Input: part model. Units: mm. Frame: model coordinates. Face numbers are marked on the shaded views. A direction names the side the tool comes from. Coordinates: 2 decimals unless noted, no trailing zeros. Loops run counter-clockwise (first coordinate to the right, second up) from the corner with the lowest first, then second, coordinate; pieces in that order, holes last.
Item 1: Pull-direction query (X, two-part tool) for the marked faces 1, 2, 3 and 4; classes: released by +X, released by -X, zero draft, split by the parting line, or undercut.
Item 2: Section C-C on x = -6. Return loops of the section in (y, z).
Item 3: Contact query for flat-ended pins moving along their axis: P1, Ø6, axis at x = 28.5, y = -37, coming from the -Z side; P2, Ø3, axis at x = -7.5, z = 42, coming from the +Y side. Output: stop coordinate, or through.
Item 4: Reachability of the marked faces 5 and 6 from +Z, -Z, +X, -X, +Y, -Y: full face, straight path, thin tool, end or side. Return the list, or none.
Item 5: Section B-B on y = 11.5. Return loops of the section in (x, z).
Item 6: Ray query, line 1 along X through (y, z) = (11.5, 58); line 2 along Y through (x, z) = (45, 51); line 3 along Z through (x, y) = (5.5, 21). Return the intervals inside material, ascending.
Item 7: Section A-A on z = 19.5. Return loops of the section in (x, y), and give its area (3 significant figures).
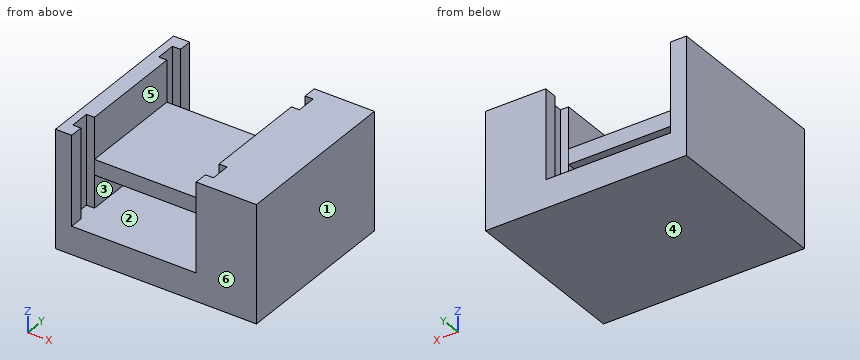
```python
from build123d import *

# Parameters (mm, degrees)
F1_DEPTH  = 17.93161
F2_DEPTH  = 75.24566
F3_W      = 80
F3_H      = 9.859875
F4_DEPTH  = 33.73
F2_FACE_W = 110
F2_FACE_H = 75.24566
F5_DEPTH  = 28.33094


with BuildPart() as f1:
    # F0 (on Top) → F1 (new body)
    with BuildSketch(Plane.XY):
        Polygon((-40, -55), (0, -55), (0, 0), (-40, 0), (-40, -33.72997), (-45.169481, -33.72997), (-45.169481, -46.42997), (-40, -46.42997), align=None)
        Polygon((0, 0), (0, -55), (40, -55), (40, -46.42997), (45.169481, -46.42997), (45.169481, -33.72997), (40, -33.72997), (40, 0), align=None)
        Polygon((-40, 0), (0, 0), (0, 55), (-40, 55), (-40, 46.42997), (-45.169481, 46.42997), (-45.169481, 33.72997), (-40, 33.72997), align=None)
        Polygon((0, 55), (0, 0), (40, 0), (40, 33.72997), (45.169481, 33.72997), (45.169481, 46.42997), (40, 46.42997), (40, 55), align=None)
        Polygon((-50.338964, -55), (-40, -55), (-40, -46.42997), (-45.169481, -46.42997), (-45.169481, -33.72997), (-40, -33.72997), (-40, 0), (-50.338964, 0), align=None)
        Polygon((40, -46.42997), (40, -55), (50.338964, -55), (50.338964, 0), (40, 0), (40, -33.72997), (45.169481, -33.72997), (45.169481, -46.42997), align=None)
        Polygon((40, 33.72997), (40, 0), (50.338964, 0), (50.338964, 55), (40, 55), (40, 46.42997), (45.169481, 46.42997), (45.169481, 33.72997), align=None)
        Polygon((-50.338964, 0), (-40, 0), (-40, 33.72997), (-45.169481, 33.72997), (-45.169481, 46.42997), (-40, 46.42997), (-40, 55), (-50.338964, 55), align=None)
    extrude(amount=F1_DEPTH)

    # F0 (on Top) → F2 (join)
    with BuildSketch(Plane.XY):
        Polygon((40, -46.42997), (40, -55), (50.338964, -55), (50.338964, 0), (40, 0), (40, -33.72997), (45.169481, -33.72997), (45.169481, -46.42997), align=None)
        Polygon((-50.338964, -55), (-40, -55), (-40, -46.42997), (-45.169481, -46.42997), (-45.169481, -33.72997), (-40, -33.72997), (-40, 0), (-50.338964, 0), align=None)
        Polygon((-50.338964, 0), (-40, 0), (-40, 33.72997), (-45.169481, 33.72997), (-45.169481, 46.42997), (-40, 46.42997), (-40, 55), (-50.338964, 55), align=None)
        Polygon((40, 33.72997), (40, 0), (50.338964, 0), (50.338964, 55), (40, 55), (40, 46.42997), (45.169481, 46.42997), (45.169481, 33.72997), align=None)
    extrude(amount=F2_DEPTH)

    # F3 (on Front) → F4 (join, symmetric)
    with BuildSketch(Plane.XZ):
        with Locations((0, 43.787974)):
            Rectangle(F3_W, F3_H)
    extrude(amount=F4_DEPTH, both=True)

    # F2_face (on face) → F5 (join)
    with BuildSketch(Plane(origin=(50.338964, 0, 37.62283), x_dir=(0, 1, 0), z_dir=(1, 0, 0))):
        Rectangle(F2_FACE_W, F2_FACE_H)
    extrude(amount=F5_DEPTH)


solid = f1.part
```
Results found:
1. face 1: released by +X
1. face 2: undercut
1. face 3: undercut
1. face 4: zero draft
2. outline: (-55, 0) - (55, 0) - (55, 17.93) - (-55, 17.93) - close; (-33.73, 38.86) - (33.73, 38.86) - (33.73, 48.72) - (-33.73, 48.72) - close
3. P1: stops at z = 0
3. P2: stops at y = 33.73
4. face 5: +Z, +Y, -Y
4. face 6: +Z, -Z, +X, -X, -Y
5. outline: (-50.34, 0) - (78.67, 0) - (78.67, 75.25) - (40, 75.25) - (40, 48.72) - (-40, 48.72) - (-40, 75.25) - (-50.34, 75.25) - close; hole (-40, 17.93) - (40, 17.93) - (40, 38.86) - (-40, 38.86) - close
6. line 1: x = -50.34 to -40, 40 to 78.67
6. line 2: y = -55 to -46.43, -33.73 to 33.73, 46.43 to 55
6. line 3: z = 0 to 17.93, 38.86 to 48.72
7. outline: (-50.34, -55) - (-40, -55) - (-40, -46.43) - (-45.17, -46.43) - (-45.17, -33.73) - (-40, -33.73) - (-40, 33.73) - (-45.17, 33.73) - (-45.17, 46.43) - (-40, 46.43) - (-40, 55) - (-50.34, 55) - close; (40, -55) - (78.67, -55) - (78.67, 55) - (40, 55) - (40, 46.43) - (45.17, 46.43) - (45.17, 33.73) - (40, 33.73) - (40, -33.73) - (45.17, -33.73) - (45.17, -46.43) - (40, -46.43) - close
7. area: 5,130 mm2
